Read the model definition and answer for the solid it produces. Units are mm, in the model's axes. Coordinates: 2 decimals unless noted, no trailing zeros. Write each loop counter-clockwise with the first axis right and the second up, starting at its lowest first coordinate (ties: lowest second). Pieces come first, ordered by that corner, then holes. Notation, with made-up numbers: (71.25, 7.5) -> (94.25, 7.5) arc R30 cw to (94.25, 30.5) -> close; hole circle Ø9 at (56.25, 73.5). An arc over 180 degrees is marked (long way). Return JSON: item names as keys, results as strings.
from build123d import *

# Parameters (mm, degrees)
SKETCH1_R           = 1.5
BOSS_EXTRUDE1_DEPTH = 3
SKETCH2_R           = 0.25
BOSS_EXTRUDE2_DEPTH = 11.5


# Read off the part's stored shape, not the designer's step: Dome1
with BuildPart() as part:
    # Sketch1 → Boss-Extrude1 (new body)
    with BuildSketch(Plane(origin=(0, 0, 0), x_dir=(1, 0, 0), z_dir=(0, 1, 0))):
        with Locations(Location((0, 0, 0), (0, 0, 270))):
            Circle(SKETCH1_R)
    extrude(amount=BOSS_EXTRUDE1_DEPTH)

    # Dome1 outline → Dome1 (revolve)
    with BuildSketch(Plane.XY):
        with BuildLine():
            Line((0, 3), (1.5, 2.999999998))
            ThreePointArc((1.5, 2.999999998), (1.060660172, 4.060660171), (0, 4.5))
            Line((0, 4.5), (0, 3))
        make_face()
    revolve(axis=Axis((0, 0, 0), (0, 1, 0)))

    # Sketch2 → Boss-Extrude2 (add)
    with BuildSketch(Plane.XZ):
        with Locations(Location((0, 0.75, 0), (0, 0, 90))):
            Circle(SKETCH2_R)
        with Locations(Location((0, -0.75, 0), (0, 0, 90))):
            Circle(SKETCH2_R)
    extrude(amount=BOSS_EXTRUDE2_DEPTH)


solid = part.part
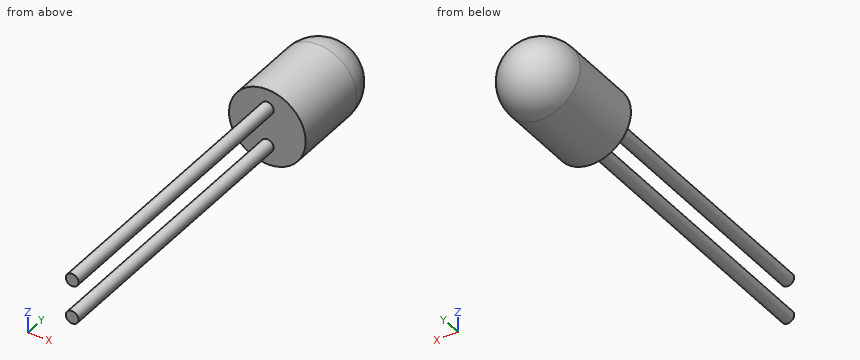
1. The part is cut by section D-D (y = 1.25). Determine the outline of the cut face in (x, z).
Taken from the geometry:
{"outline": "circle Ø3 at (0, 0)"}
2. The part is cut by section B-B (y = -10.25). Determine the outline of the cut face in (x, z), then the cut area to 3 significant figures.
Taken from the geometry:
{"outline": "circle Ø0.5 at (0, -0.75); circle Ø0.5 at (0, 0.75)", "area": "0.393 mm2"}
3. The part is cut by section C-C (z = 0.7). Determine the outline of the cut face in (x, y), then the cut area to 3 significant figures.
Taken from the geometry:
{"outline": "(-1.33, 0) -> (-0.24, 0) -> (-0.24, -11.5) -> (0.24, -11.5) -> (0.24, 0) -> (1.33, 0) -> (1.33, 3) arc R1.33 ccw to (-1.33, 3) -> close", "area": "16.4 mm2"}
4. Consider L1, parallel to X at y = 2.25, z = -0.1; L2, parallel to Y at x = 0, z = 0.05; L3, parallel to Z at x = 0.2, y = -7. Determine where each line is inside the solid, lowest interval first.
Taken from the geometry:
{"L1": "x = -1.5 to 1.5", "L2": "y = 0 to 4.5", "L3": "z = -0.9 to -0.6, 0.6 to 0.9"}
5. The part is cut by section A-A (x = 0). Determine the outline of the cut face in (y, z), then the cut area to 3 significant figures.
Taken from the geometry:
{"outline": "(-11.5, -1) -> (0, -1) -> (0, -1.5) -> (3, -1.5) arc R1.5 ccw to (3, 1.5) -> (0, 1.5) -> (0, 1) -> (-11.5, 1) -> (-11.5, 0.5) -> (0, 0.5) -> (0, -0.5) -> (-11.5, -0.5) -> close", "area": "24.0 mm2"}
6. A flat-ended cylindrical pin translates along its axis: pin 1 Ø1.5 at (x, z) = (-0.5, 0.5) entering from -Y. Find the tip coordinate at first contact, or state that the pin passes through.
Taken from the geometry:
{"pin 1": "stops at y = -11.5"}
